```python
from build123d import *

# Parameters (mm, degrees)
F0_R     = 12.7
F1_DEPTH = 25.4
F3_DEPTH = 25.4
F4_R     = 12.7


with BuildPart() as f1:
    # F0 (on Front) → F1 (new body)
    with BuildSketch(Plane.XZ):
        with BuildLine():
            Line((58.1624929965, -35.6950488269), (-29.1996338754, 23.4392795148))
            ThreePointArc((-29.1996338754, 23.4392795148), (-55.3437663352, 24.841550486), (-68.8375070035, 2.4049511731))
            Line((-68.8375070035, 2.4049511731), (-68.8375070035, -48.3950488269))
            Line((-68.8375070035, -48.3950488269), (58.1624929965, -48.3950488269))
            Line((58.1624929965, -48.3950488269), (58.1624929965, -35.6950488269))
        make_face()
        with Locations((-43.4375070035, 2.4049511731)):
            Circle(F0_R, mode=Mode.SUBTRACT)
    extrude(amount=F1_DEPTH)

    # F2 (on face) → F3 (join)
    with BuildSketch(Plane.XZ.offset(25.4)):
        with BuildLine():
            Line((-18.151617463, -35.6950488269), (-18.151617463, 0))
            ThreePointArc((-18.151617463, 0), (-20.4618261667, 13.2344520888), (-29.1996338754, 23.4392795148))
            ThreePointArc((-29.1996338754, 23.4392795148), (-55.3437663352, 24.841550486), (-68.8375070035, 2.4049511731))
            Line((-68.8375070035, 2.4049511731), (-68.8375070035, -35.6950488269))
            Line((-68.8375070035, -35.6950488269), (-68.8375070035, -48.3950488269))
            Line((-68.8375070035, -48.3950488269), (58.1624929965, -48.3950488269))
            Line((58.1624929965, -48.3950488269), (58.1624929965, -35.6950488269))
            Line((58.1624929965, -35.6950488269), (-18.151617463, -35.6950488269))
        make_face()
        with BuildLine():
            ThreePointArc((-30.9672941002, 0), (-56.0799297119, 3.6129031852), (-30.7375070035, 2.4049511731))
            ThreePointArc((-30.7375070035, 2.4049511731), (-30.7950842952, 1.1969991609), (-30.9672941002, 0))
        make_face(mode=Mode.SUBTRACT)
    extrude(amount=F3_DEPTH)

    # F4
    f4_edges = [f1.edges().sort_by_distance(p)[0] for p in [
        (58.162493, -50.8, -42.045049),
    ]]
    fillet(f4_edges, radius=F4_R)


solid = f1.part
```
CAD build for the part. Positions are in the model's coordinates, mm. Coordinates: 2 decimals unless noted, no trailing zeros. Write each loop counter-clockwise with the first axis right and the second up, starting at its lowest first coordinate (ties: lowest second). Pieces come first, ordered by that corner, then holes. Notation, with made-up numbers: (62.25, -39.75) -> (94.25, -39.75) arc R14 ccw to (94.25, -33.75) -> close; hole circle Ø7 at (50, 84). An arc over 180 degrees is marked (long way). Return JSON: item names as keys, results as strings. Group by question number.
Q1. Drill centre lines: line 1 (X direction, y = -44, z = 2.5); line 2 (Z direction, x = 47, y = -34.5); line 3 (X direction, y = -39.5, z = -4). Where is each one in solid material? Low to high.
Q2. Cut at B-B, the plane z = 4.5. Give the cut face in (x, y).
Q3. Pull direction Z, two halves, no side cores. Call faces 1 (the face through (-6, -25, -48.395)), 2 (the face through (-20, 0, -18)), 3 (the face through (15.09, -12.52, -6.54)), 4 (the face through (-18.152, -38, -18)): released by +Z, released by -Z, zero draft, split by the parting line, or undercut.
Q4. Flat gauge pins, fed straight in: pin 1 (3 mm diameter, centred on x = 42.5, y = -7, fed in from +Z); pin 2 (8 mm diameter, centred on x = 28, y = -20, fed in from +Z); pin 3 (10 mm diameter, centred on y = -12, z = -27.5, fed in from +X). Where does each tip first touch, or does it go through?
Q5. Cut at D-D, the plane y = -9.5. Give the cut face in (x, z), then the cut area to 3 significant figures.
Q6. Cut at A-A, the plane y = -34. Give the cut face in (x, z).
Q7. Cut at C-C, the plane x = 3. Give the cut face in (y, z), then the cut area to 3 significant figures.
Returned:
{
 "1": {"line 1": "x = -68.84 to -56.14, -30.74 to -18.04", "line 2": "z = -48.4 to -35.7", "line 3": "x = -68.84 to -54.4, -32.47 to -18.15"},
 "2": {"outline": "(-68.75, -50.8) -> (-55.96, -50.8) -> (-55.96, 0) -> (-68.75, 0) -> close; (-30.91, -50.8) -> (-18.12, -50.8) -> (-18.12, -25.4) -> (-1.22, -25.4) -> (-1.22, 0) -> (-30.91, 0) -> close"},
 "3": {"face 1": "released by -Z", "face 2": "zero draft", "face 3": "released by +Z", "face 4": "undercut"},
 "4": {"pin 1": "stops at z = -24.08", "pin 2": "stops at z = -12.57", "pin 3": "stops at x = 53.44"},
 "5": {"outline": "(-68.84, -48.4) -> (58.16, -48.4) -> (58.16, -35.7) -> (-29.2, 23.44) arc R25.4 ccw to (-68.84, 2.4) -> close; hole circle Ø25.4 at (-43.44, 2.4)", "area": "6,050 mm2"},
 "6": {"outline": "(-68.84, -48.4) -> (58.16, -48.4) -> (58.16, -35.7) -> (-18.15, -35.7) -> (-18.15, 0) arc R25.4 ccw (long way) to (-68.84, 2.4) -> close; hole circle Ø25.4 at (-43.44, 2.4)"},
 "7": {"outline": "(-50.8, -48.4) -> (0, -48.4) -> (0, 1.64) -> (-25.4, 1.64) -> (-25.4, -35.7) -> (-50.8, -35.7) -> close", "area": "1,590 mm2"}
}
